Autodesk Fusion 360 part; units mm, degrees
sketch "Sketch1" plane through (0, 0, 0) normal (0, 0, 1) x (1, 0, 0)
  line L0 (0, 0) -> (0, 500)
  line L1 (0, 500) -> (350, 500)
  line L2 (350, 500) -> (350, 0)
  line L3 (350, 0) -> (0, 0)
  dimension "d6" = 500
  dimension "d7" = 350
  dimension "d8" = 500
  dimension "d9" = 350
extrude "Extrude1" add sketch "Sketch1" along normal blind 21
sketch "Sketch2" plane through (0, 0, 21) normal (0, 0, 1) x (-1, 0, 0)
  line L0 (-350, 0) -> (-350, -500)
  line L1 (-350, -500) -> (0, -500)
  line L2 (0, -500) -> (0, 0)
  line L3 (0, 0) -> (-350, 0)
  line L4 (0, 0) -> (-20, 0)
  line L5 (-350, 0) -> (-330, 0)
  line L6 (-330, 0) -> (-330, -500)
  line L7 (-20, 0) -> (-20, -500)
  line L8 (-20, -500) -> (-110, -500)
  line L9 (-110, -500) -> (-130, -500)
  line L10 (-130, -500) -> (-220, -500)
  line L11 (-220, -500) -> (-240, -500)
  line L12 (-240, -500) -> (-330, -500)
  line L13 (-110, -500) -> (-110, 0)
  line L14 (-130, -500) -> (-130, 0)
  line L15 (-220, -500) -> (-220, 0)
  line L16 (-240, -500) -> (-240, 0)
  line L17 (0, 0) -> (0, -95)
  line L18 (0, -500) -> (0, -405)
  line L19 (0, -405) -> (-350, -405)
  line L20 (0, -95) -> (-350, -95)
  line L21 (0, -405) -> (0, -315)
  line L22 (0, -315) -> (0, -295)
  line L23 (0, -295) -> (0, -205)
  line L24 (0, -205) -> (0, -185)
  line L25 (0, -185) -> (0, -95)
  line L26 (0, -185) -> (-350, -185)
  line L27 (0, -205) -> (-350, -205)
  line L28 (0, -295) -> (-350, -295)
  line L29 (0, -315) -> (-350, -315)
  dimension "d13" = 20
  dimension "d14" = 500
  dimension "d16" = 90
  dimension "d19" = 20
  dimension "d27" = 95
  dimension "d28" = 95
  dimension "d29" = 350
  dimension "d31" = 90
  dimension "d32" = 20
  dimension "d34" = 90
  dimension "d35" = 20
extrude "Extrude2" cut sketch "Sketch2" against normal blind 10 contours L6 L16 L20 L26 | L6 L16 L27 L28 | L14 L15 L20 L26 | L6 L16 L19 L29 | L14 L15 L27 L28 | L7 L13 L20 L26 | L14 L15 L19 L29 | L7 L13 L27 L28 | L7 L13 L19 L29
sketch "Sketch3" plane through (0, 0, 21) normal (0, 0, 1) x (-1, 0, 0)
  line L0 (-330, -95) -> (-240, -95)
  line L1 (-240, -95) -> (-240, -185)
  line L2 (-240, -185) -> (-330, -185)
  line L3 (-330, -185) -> (-330, -95)
  line L4 (-130, -205) -> (-130, -295)
  line L5 (-130, -295) -> (-220, -295)
  line L6 (-220, -295) -> (-220, -205)
  line L7 (-220, -205) -> (-130, -205)
  line L8 (-110, -405) -> (-110, -315)
  line L9 (-110, -315) -> (-20, -315)
  line L10 (-20, -315) -> (-20, -405)
  line L11 (-20, -405) -> (-110, -405)
  line L12 (-110, -295) -> (-110, -205)
  line L13 (-110, -205) -> (-20, -205)
  line L14 (-20, -205) -> (-20, -295)
  line L15 (-20, -295) -> (-110, -295)
  line L16 (-130, -95) -> (-130, -185)
  line L17 (-130, -185) -> (-220, -185)
  line L18 (-220, -185) -> (-220, -95)
  line L19 (-220, -95) -> (-130, -95)
  line L20 (-330, -205) -> (-240, -205)
  line L21 (-240, -205) -> (-240, -295)
  line L22 (-240, -295) -> (-330, -295)
  line L23 (-330, -295) -> (-330, -205)
  line L24 (-130, -315) -> (-130, -405)
  line L25 (-130, -405) -> (-220, -405)
  line L26 (-220, -405) -> (-220, -315)
  line L27 (-220, -315) -> (-130, -315)
  line L28 (-330, -315) -> (-240, -315)
  line L29 (-240, -315) -> (-240, -405)
  line L30 (-240, -405) -> (-330, -405)
  line L31 (-330, -405) -> (-330, -315)
  line L32 (-110, -185) -> (-110, -95)
  line L33 (-110, -95) -> (-20, -95)
  line L34 (-20, -95) -> (-20, -185)
  line L35 (-20, -185) -> (-110, -185)
  line L36 (0, 0) -> (-175, 0)
  circle A0 centre (-175, -50) radius 5.5
  circle A1 centre (-208, -50) radius 5.5
  circle A2 centre (-241, -50) radius 5.5
  circle A3 centre (-142, -50) radius 5.5
  circle A4 centre (-109, -50) radius 5.5
  line L37 (0, -500) -> (-175, -500)
  circle A5 centre (-142, -450) radius 5.5
  circle A6 centre (-109, -450) radius 5.5
  circle A7 centre (-208, -450) radius 5.5
  circle A8 centre (-175, -450) radius 5.5
  circle A9 centre (-241, -450) radius 5.5
  line L38 (-350, 0) -> (-350, -500)
  line L39 (-350, -500) -> (0, -500)
  line L40 (0, -500) -> (0, 0)
  line L41 (0, 0) -> (-350, 0)
  dimension "d43" = 175
  dimension "d44" = 50
  dimension "d46" = 33
  dimension "d55" = 11
  dimension "d56" = 175
  dimension "d57" = 50
  dimension "d60" = 33
  dimension "d64" = 11
extrude "Extrude3" cut sketch "Sketch3" against normal blind 11 contours A0 | A1 | A2 | A3 | A4 | A5 | A6 | A7 | A8 | A9
sketch "Sketch5" plane through (0, 0, 21) normal (0, 0, 1) x (-1, 0, 0)
  circle A0 centre (-175, -50) radius 5.5
  circle A1 centre (-208, -450) radius 5.5
  circle A2 centre (-109, -450) radius 5.5
  circle A3 centre (-241, -450) radius 5.5
  circle A4 centre (-208, -50) radius 5.5
  circle A5 centre (-142, -50) radius 5.5
  circle A6 centre (-175, -450) radius 5.5
  circle A7 centre (-142, -450) radius 5.5
  circle A8 centre (-109, -50) radius 5.5
  circle A9 centre (-241, -50) radius 5.5
  line L0 (-110, -185) -> (-110, -95)
  line L1 (-110, -95) -> (-20, -95)
  line L2 (-20, -95) -> (-20, -185)
  line L3 (-20, -185) -> (-110, -185)
  line L4 (-330, -315) -> (-240, -315)
  line L5 (-240, -315) -> (-240, -405)
  line L6 (-240, -405) -> (-330, -405)
  line L7 (-330, -405) -> (-330, -315)
  line L8 (-130, -315) -> (-130, -405)
  line L9 (-130, -405) -> (-220, -405)
  line L10 (-220, -405) -> (-220, -315)
  line L11 (-220, -315) -> (-130, -315)
  line L12 (-330, -205) -> (-240, -205)
  line L13 (-240, -205) -> (-240, -295)
  line L14 (-240, -295) -> (-330, -295)
  line L15 (-330, -295) -> (-330, -205)
  line L16 (-130, -95) -> (-130, -185)
  line L17 (-130, -185) -> (-220, -185)
  line L18 (-220, -185) -> (-220, -95)
  line L19 (-220, -95) -> (-130, -95)
  line L20 (-110, -295) -> (-110, -205)
  line L21 (-110, -205) -> (-20, -205)
  line L22 (-20, -205) -> (-20, -295)
  line L23 (-20, -295) -> (-110, -295)
  line L24 (-110, -405) -> (-110, -315)
  line L25 (-110, -315) -> (-20, -315)
  line L26 (-20, -315) -> (-20, -405)
  line L27 (-20, -405) -> (-110, -405)
  line L28 (-130, -205) -> (-130, -295)
  line L29 (-130, -295) -> (-220, -295)
  line L30 (-220, -295) -> (-220, -205)
  line L31 (-220, -205) -> (-130, -205)
  line L32 (-330, -95) -> (-240, -95)
  line L33 (-240, -95) -> (-240, -185)
  line L34 (-240, -185) -> (-330, -185)
  line L35 (-330, -185) -> (-330, -95)
  line L36 (-350, 0) -> (-350, -500)
  line L37 (-350, -500) -> (0, -500)
  line L38 (0, -500) -> (0, 0)
  line L39 (0, 0) -> (-350, 0)
equation "lengd = 500 mm"
equation "breydd = 350 mm"
equation "dypt_holfa = 10 mm"
equation "veggir = 20 mm"
equation "d6 = lengd"
equation "d7 = breydd"
equation "d8 = lengd"
equation "d9 = breydd"
equation "d13 = veggir"
equation "d14 = lengd"
equation "d16 = ( breydd - veggir ) / 3 - veggir"
equation "d19 = veggir"
equation "d27 = ( ( lengd - breydd ) / 2 ) + veggir"
equation "d28 = ( ( lengd - breydd ) / 2 ) + veggir"
equation "d29 = breydd"
equation "d31 = ( ( breydd - veggir ) / 3 ) - veggir"
equation "d32 = veggir"
equation "d34 = ( ( breydd - veggir ) / 3 ) - veggir"
equation "d35 = veggir"
equation "renna_stiga = 5 mm"
equation "renna_breydd = 5 mm"
equation "d43 = breydd / 2"
equation "d44 = ( lengd / 10 )"
equation "d46 = Linear Dimension-4"
equation "d55 = Diameter Dimension-3"
equation "d56 = breydd / 2"
equation "d57 = lengd / 10"
equation "d60 = Linear Dimension-8"
equation "d64 = Diameter Dimension-4"
Read the model definition and answer for the solid it produces. Units are mm, in the model's axes. Round coordinates to 2 decimals unless told otherwise and drop trailing zeros. Order: outer loops, then holes, each group sorted by start corner. A loop starts at its lowest first (then second) coordinate and runs counter-clockwise, first axis right, second up.
1) The part is cut by section D-D on y = 101. Write down the section's boundary in (x, z).
2) The part is cut by section A-A on y = 50. Write down the section's boundary in (x, z), plus the area to 4 significant figures.
3) The part is cut by section C-C on x = 95. Write down the section's boundary in (y, z).
4) Straight lines are drawn through the part: L1, parallel to X at y = 270, z = 19.5; L2, parallel to Y at x = 142, z = 18; L3, parallel to X at y = 50, z = 14. For each, find the intervals that lie inside material, in ascending order.
5) The mould has two halves that part along Y. Classify faces 1 (the face through (173, 254, 0)), 2 (the face through (174, 205, 16)): released by +Y, released by -Y, zero draft, split by the parting line, or undercut.
6) The part is cut by section B-B on x = 142. Write down the section's boundary in (y, z).
Resolved:
1. outline: (0, 0) - (350, 0) - (350, 21) - (330, 21) - (330, 11) - (240, 11) - (240, 21) - (220, 21) - (220, 11) - (130, 11) - (130, 21) - (110, 21) - (110, 11) - (20, 11) - (20, 21) - (0, 21) - close
2. outline: (0, 0) - (350, 0) - (350, 21) - (246.5, 21) - (246.5, 10) - (235.5, 10) - (235.5, 21) - (213.5, 21) - (213.5, 10) - (202.5, 10) - (202.5, 21) - (180.5, 21) - (180.5, 10) - (169.5, 10) - (169.5, 21) - (147.5, 21) - (147.5, 10) - (136.5, 10) - (136.5, 21) - (114.5, 21) - (114.5, 10) - (103.5, 10) - (103.5, 21) - (0, 21) - close
2. area: 6,745 mm2
3. outline: (0, 0) - (500, 0) - (500, 21) - (405, 21) - (405, 11) - (315, 11) - (315, 21) - (295, 21) - (295, 11) - (205, 11) - (205, 21) - (185, 21) - (185, 11) - (95, 11) - (95, 21) - (0, 21) - close
4. L1: x = 0 to 20, 110 to 130, 220 to 240, 330 to 350
4. L2: y = 0 to 44.5, 55.5 to 95, 185 to 205, 295 to 315, 405 to 444.5, 455.5 to 500
4. L3: x = 0 to 103.5, 114.5 to 136.5, 147.5 to 169.5, 180.5 to 202.5, 213.5 to 235.5, 246.5 to 350
5. face 1: zero draft
5. face 2: undercut
6. outline: (0, 0) - (500, 0) - (500, 21) - (455.5, 21) - (455.5, 10) - (444.5, 10) - (444.5, 21) - (405, 21) - (405, 11) - (315, 11) - (315, 21) - (295, 21) - (295, 11) - (205, 11) - (205, 21) - (185, 21) - (185, 11) - (95, 11) - (95, 21) - (55.5, 21) - (55.5, 10) - (44.5, 10) - (44.5, 21) - (0, 21) - close
